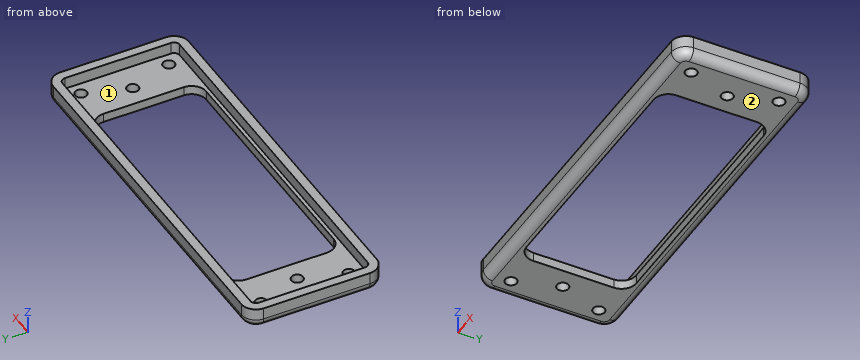
```python
from build123d import *

# Parameters (mm, degrees)
F1_DEPTH = 2.5
F2_R     = 1.6
F3_DEPTH = 2.501
F5_DEPTH = 3.25
F6_R     = 2.5


with BuildPart() as f1:
    # F0 (on Top) → F1 (new body)
    with BuildSketch(Plane.XY):
        with BuildLine():
            ThreePointArc((52, 14.5), (50.828427, 17.328427), (48, 18.5))
            Line((48, 18.5), (-48, 18.5))
            ThreePointArc((-48, 18.5), (-50.828427, 17.328427), (-52, 14.5))
            Line((-52, 14.5), (-52, -14.5))
            ThreePointArc((-52, -14.5), (-50.828427, -17.328427), (-48, -18.5))
            Line((-48, -18.5), (48, -18.5))
            ThreePointArc((48, -18.5), (50.828427, -17.328427), (52, -14.5))
            Line((52, -14.5), (52, 14.5))
        make_face()
        with BuildLine():
            Line((-32.5, 15), (32.5, 15))
            ThreePointArc((32.5, 15), (35.328427, 13.828427), (36.5, 11))
            Line((36.5, 11), (36.5, -11))
            ThreePointArc((36.5, -11), (35.328427, -13.828427), (32.5, -15))
            Line((32.5, -15), (-32.5, -15))
            ThreePointArc((-32.5, -15), (-35.328427, -13.828427), (-36.5, -11))
            Line((-36.5, -11), (-36.5, 11))
            ThreePointArc((-36.5, 11), (-35.328427, 13.828427), (-32.5, 15))
        make_face(mode=Mode.SUBTRACT)
    extrude(amount=F1_DEPTH)

    # F2 (on face) → F3 (cut, through all)
    with BuildSketch(Plane.XY.offset(2.5)):
        with Locations((-46, 12)):
            Circle(F2_R)
        with Locations((46, 12)):
            Circle(F2_R)
        with Locations((46, -12)):
            Circle(F2_R)
        with Locations((-46, -12)):
            Circle(F2_R)
        with Locations((-42, 0)):
            Circle(F2_R)
        with Locations((42, 0)):
            Circle(F2_R)
    extrude(amount=-F3_DEPTH, mode=Mode.SUBTRACT)

    # F4 (on face) → F5 (join)
    with BuildSketch(Plane.XY.offset(2.5)):
        with BuildLine():
            Line((48, 18.5), (-48, 18.5))
            ThreePointArc((-48, 18.5), (-50.828427, 17.328427), (-52, 14.5))
            Line((-52, 14.5), (-52, -14.5))
            ThreePointArc((-52, -14.5), (-50.828427, -17.328427), (-48, -18.5))
            Line((-48, -18.5), (48, -18.5))
            ThreePointArc((48, -18.5), (50.828427, -17.328427), (52, -14.5))
            Line((52, -14.5), (52, 14.5))
            ThreePointArc((52, 14.5), (50.828427, 17.328427), (48, 18.5))
        make_face()
        with BuildLine():
            Line((-49.5, -14.5), (-49.5, 14.5))
            ThreePointArc((-49.5, 14.5), (-49.06066, 15.56066), (-48, 16))
            Line((-48, 16), (48, 16))
            ThreePointArc((48, 16), (49.06066, 15.56066), (49.5, 14.5))
            Line((49.5, 14.5), (49.5, -14.5))
            ThreePointArc((49.5, -14.5), (49.06066, -15.56066), (48, -16))
            Line((48, -16), (-48, -16))
            ThreePointArc((-48, -16), (-49.06066, -15.56066), (-49.5, -14.5))
        make_face(mode=Mode.SUBTRACT)
    extrude(amount=F5_DEPTH)

    # F6
    f6_edges = [f1.edges().sort_by_distance(p)[0] for p in [
        (-50.828427, 17.328427, 0),
        (0, 18.5, 0),
        (-52, 0, 0),
        (-50.828427, -17.328427, 0),
        (0, -18.5, 0),
        (50.828427, -17.328427, 0),
        (52, 0, 0),
        (50.828427, 17.328427, 0),
    ]]
    fillet(f6_edges, radius=F6_R)


solid = f1.part
```
Verification items for the finished model (mm, model axes). Face numbers are marked on the shaded views. Give positions to 0.01 mm unless a question says otherwise; leave off trailing zeros. Order: outer loops, then holes, each group sorted by start corner. A loop starts at its lowest first (then second) coordinate and runs counter-clockwise, first axis right, second up. Notation, with made-up numbers: M 81.25,73.5 L 121.25,73.5 A34 cw 121.25,105.5 Z; hole C 1.25,75 d5. An arc over 180 degrees is marked long. Return JSON: item names as keys, results as strings. Group by question number.
1) Section check A-A on y = 0. Record the cut outline in (x, z), and give its area (3 significant figures).
2) Go/stop test with flat-tipped pins: pin 1 Ø1.5 at (y, z) = (-14.5, 1) entering from +X; pin 2 Ø3.5 at (x, y) = (-46, -12) entering from +Z; pin 3 Ø3 at (x, z) = (-19, 0.5) entering from -Y. Record where each tip stops, or that it passes through.
3) Section check B-B on y = -7.5. Record the cut outline in (x, z), and give its area (3 significant figures).
4) Section check D-D on z = 3.85. Record the cut outline in (x, y).
5) Scan lines: line 1 (Y direction, x = 36.5, z = 3.3); line 2 (Y direction, x = 46, z = 0.8); line 3 (X direction, y = -8.5, z = 3.4). Record each from-to range of solid material in increasing order.
6) Mould release check, pull along X, two halves, no side actions. Record for the marked faces 1 and 2: pulls with the +X half, pulls with the -X half, needs draft (parallel to the pull), parting line crosses it, or undercut.
7) Section check C-C on x = -28.5. Record the cut outline in (y, z).
Answer block:
{
 "1": {"outline": "M -52,2.5 A2.5 ccw -49.5,0 L -43.6,0 L -43.6,2.5 L -49.5,2.5 L -49.5,5.75 L -52,5.75 Z; M -40.4,0 L -36.5,0 L -36.5,2.5 L -40.4,2.5 Z; M 36.5,0 L 40.4,0 L 40.4,2.5 L 36.5,2.5 Z; M 43.6,0 L 49.5,0 A2.5 ccw 52,2.5 L 52,5.75 L 49.5,5.75 L 49.5,2.5 L 43.6,2.5 Z", "area": "75.1 mm^2"},
 "2": {"pin 1": "stops at x = 51.88", "pin 2": "stops at z = 2.5", "pin 3": "stops at y = -18.45"},
 "3": {"outline": "M -52,2.5 A2.5 ccw -49.5,0 L -36.5,0 L -36.5,2.5 L -49.5,2.5 L -49.5,5.75 L -52,5.75 Z; M 36.5,0 L 49.5,0 A2.5 ccw 52,2.5 L 52,5.75 L 49.5,5.75 L 49.5,2.5 L 36.5,2.5 Z", "area": "91.1 mm^2"},
 "4": {"outline": "M -52,-14.5 A4 ccw -48,-18.5 L 48,-18.5 A4 ccw 52,-14.5 L 52,14.5 A4 ccw 48,18.5 L -48,18.5 A4 ccw -52,14.5 Z; hole M -49.5,-14.5 A1.5 ccw -48,-16 L 48,-16 A1.5 ccw 49.5,-14.5 L 49.5,14.5 A1.5 ccw 48,16 L -48,16 A1.5 ccw -49.5,14.5 Z"},
 "5": {"line 1": "y = -18.5 to -16, 16 to 18.5", "line 2": "y = -17.83 to -13.6, -10.4 to 10.4, 13.6 to 17.83", "line 3": "x = -52 to -49.5, 49.5 to 52"},
 "6": {"face 1": "undercut", "face 2": "needs draft"},
 "7": {"outline": "M -18.5,2.5 A2.5 ccw -16,0 L -15,0 L -15,2.5 L -16,2.5 L -16,5.75 L -18.5,5.75 Z; M 15,0 L 16,0 A2.5 ccw 18.5,2.5 L 18.5,5.75 L 16,5.75 L 16,2.5 L 15,2.5 Z"}
}
